from build123d import *

# Parameters (mm, degrees)
F1_DEPTH = 10
F3_DEPTH = 5
F4_R     = 1.5
F5_R     = 3
F7_DEPTH = 3
F10_R    = 2
F11_R    = 2.99999


# Not quite as in the source:
# - a fillet or chamfer is up to 0.001 mm smaller than in the source, because OpenCascade refuses the exact size


with BuildPart() as f1:
    # F0 (on Top) → F1 (new body, symmetric)
    with BuildSketch(Plane.XY):
        Polygon((0, 0), (-35, 0), (-35, 15), (-39, 15), (-39, -4), (61, -4), (61, 13.4), (74, 13.4), (74, 36.8), (60, 36.8), (60, 32.8), (70, 32.8), (70, 17.4), (47, 17.4), (47, 13.4), (57, 13.4), (57, 0), (4, 0), (4, 13.4), (14, 13.4), (14, 17.4), (4, 17.4), (4, 32.8), (14, 32.8), (14, 36.8), (0, 36.8), align=None)
    extrude(amount=F1_DEPTH, both=True)

    # F2 (on Top) → F3 (join, symmetric)
    with BuildSketch(Plane.XY):
        Polygon((60, 43.8), (60, 36.8), (63, 36.8), (63, 40.8), (67, 40.8), (67, 43.8), align=None)
        Polygon((-43, 12), (-39, 12), (-39, 15), (-46, 15), (-46, 8), (-43, 8), align=None)
    extrude(amount=F3_DEPTH, both=True)

    # F4
    f4_edges = [f1.edges().sort_by_distance(p)[0] for p in [
        (-35, 0, 0),
        (4, 0, 0),
        (4, 17.4, 0),
        (63, 36.8, 0),
        (63, 40.8, 0),
        (4, 32.8, 0),
        (4, 13.4, 0),
        (70, 17.4, 0),
        (57, 0, 0),
        (70, 32.8, 0),
        (57, 13.4, 0),
        (-39, 12, 0),
        (-43, 12, 0),
        (0, 0, 0),
    ]]
    fillet(f4_edges, radius=F4_R)

    # F5
    f5_edges = [f1.edges().sort_by_distance(p)[0] for p in [
        (-39, -4, 0),
        (61, -4, 0),
        (74, 13.4, 0),
        (74, 36.8, 0),
        (60, 43.8, 0),
        (-46, 15, 0),
        (0, 36.8, 0),
        (-44.5, 8, 5),
        (67, 42.3, 5),
        (-44.5, 8, -5),
        (67, 42.3, -5),
    ]]
    fillet(f5_edges, radius=F5_R)

    # F6 (on Top) → F7 (join, symmetric)
    with BuildSketch(Plane.XY):
        Polygon((-11, -8), (-0.5, -8), (-0.5, -4), (-35.5, -4), (-35.5, -8), (-25, -8), (-25, -4.5), (-11, -4.5), align=None)
    extrude(amount=F7_DEPTH, both=True)

    # F8 (on Top) → F9 (revolve, cut)
    with BuildSketch(Plane.XY):
        Polygon((-18, -4.5), (-15.9, -4.5), (-15.9, -2), (-13.75, -2), (-13.75, 0), (-18, 0), align=None)
    revolve(axis=Axis((-18, 1.7481091395, 0), (0, 1, 0)), mode=Mode.SUBTRACT)

    # F10
    f10_edges = [f1.edges().sort_by_distance(p)[0] for p in [
        (-39, 15, -7.5),
        (-39, 15, 7.5),
    ]]
    fillet(f10_edges, radius=F10_R)

    # F11 (radius 3 in the source; OpenCascade refuses exactly that, so slightly less here)
    f11_edges = [f1.edges().sort_by_distance(p)[0] for p in [
        (-0.5, -6, -3),
        (-0.5, -6, 3),
    ]]
    fillet(f11_edges, radius=F11_R)


solid = f1.part
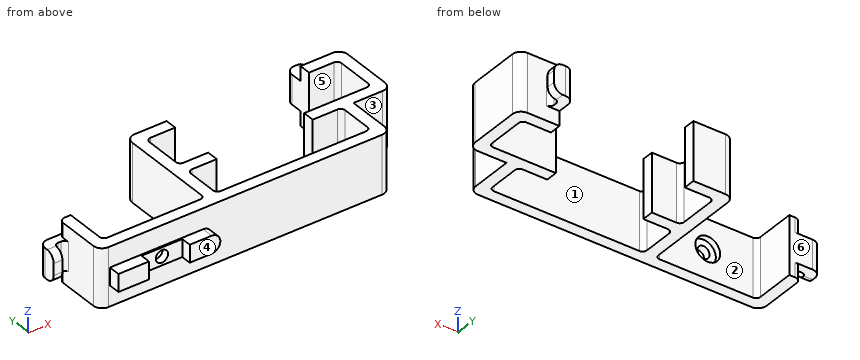
Geometry check sheet. Reference: the model listing, model coordinates, mm. Face numbers are marked on the shaded views. A direction names the side the tool comes from. Coordinates: 2 decimals unless noted, no trailing zeros. Loops run counter-clockwise (first coordinate to the right, second up) from the corner with the lowest first, then second, coordinate; pieces in that order, holes last. Notation, with made-up numbers: (-15, 22.5) - (10, 22.5) arc R21 cw to (10, 31.5) - close; hole circle Ø1 at (43, 53.25). An arc over 180 degrees is marked (long way). Use one line per item in the form item = value. Start each with the question number.
Item 1: Tool access check on the marked faces 1, 2 and 3. Record the directions out of +Z, -Z, +X, -X, +Y, -Y that give a thin tool (end or side, any length) a straight path to the whole face; none if there is none.
Item 2: Section check D-D, the plane x = -18. Enter the section's corners in (y, z), and give its area (3 significant figures).
Item 3: Section check C-C, the plane x = 9. Enter the section's corners in (y, z), and give its area (3 significant figures).
Item 4: Section check A-A, the plane x = 52. Enter the section's corners in (y, z).
Item 5: Thickness scan on probe 1 along X at (y, z) = (2, -1); probe 2 along X at (y, z) = (9, 0); probe 3 along Z at (x, y) = (-18, -3.15). Record the ranges inside material, lowest first.
Item 6: Gauge pin test, flat ends, axial feed: pin 1 (6 mm diameter, centred on x = 36.5, z = -0.5, fed in from +Y); pin 2 (11 mm diameter, centred on x = -18, z = 0, fed in from -Y); pin 3 (12 mm diameter, centred on y = -1.5, z = -2, fed in from +X). Record the tip position at first contact, or that the pin passes through.
Item 7: Section check B-B, the plane y = 25. Enter the section's corners in (x, z), and give its area (3 significant figures).
Item 8: Mould release check, pull along Y, two halves, no side actions. Record for the marked faces 4, 5 and 6: +Y half, -Y half, draft (parallel to the pull), parting line (faces both ways), or undercut.
Computed:
q1.face_1 = +Z, -Z
q1.face_2 = +Z, -Z, +Y
q1.face_3 = +Z, -Z, +X, -Y
q2.outline = (-4.5, -3) - (-4, -3) - (-4, -10) - (0, -10) - (0, -4.25) - (-2, -4.25) - (-2, -2.1) - (-4.5, -2.1) - close; (-4.5, 2.1) - (-2, 2.1) - (-2, 4.25) - (0, 4.25) - (0, 10) - (-4, 10) - (-4, 3) - (-4.5, 3) - close
q2.area = 55.5 mm2
q3.outline = (-4, -10) - (0, -10) - (0, 10) - (-4, 10) - close; (13.4, -10) - (17.4, -10) - (17.4, 10) - (13.4, 10) - close; (32.8, -10) - (36.8, -10) - (36.8, 10) - (32.8, 10) - close
q3.area = 240 mm2
q4.outline = (-4, -10) - (0, -10) - (0, 10) - (-4, 10) - close; (13.4, -10) - (17.4, -10) - (17.4, 10) - (13.4, 10) - close
q5.probe_1 = -39 to -35, 0 to 4, 57 to 61
q5.probe_2 = -46 to -43, -39 to -35, 0 to 4, 57 to 61
q5.probe_3 = -10 to -2.1, 2.1 to 10
q6.pin_1 = 0
q6.pin_2 = -4.5
q6.pin_3 = 61
q7.outline = (0, -10) - (4, -10) - (4, 10) - (0, 10) - close; (70, -10) - (74, -10) - (74, 10) - (70, 10) - close
q7.area = 160 mm2
q8.face_4 = -Y half
q8.face_5 = undercut
q8.face_6 = +Y half
